Geometry check sheet. Reference: the model listing, model coordinates, mm. Face numbers are marked on the shaded views. A direction names the side the tool comes from. Round coordinates to 2 decimals unless told otherwise and drop trailing zeros. Order: outer loops, then holes, each group sorted by start corner. A loop starts at its lowest first (then second) coordinate and runs counter-clockwise, first axis right, second up. Notation, with made-up numbers: M 4,82.5 L 25,82.5 A18 ccw 25,116.5 Z; hole C 37,26.25 d1. An arc over 180 degrees is marked long. Return JSON: item names as keys, results as strings. Group by question number.
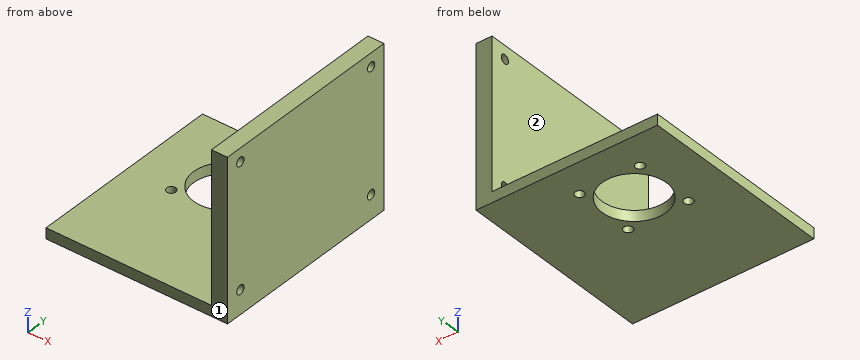
Solid Edge part; units mm, degrees
sketch "Sketch1" plane through (0, 0, 8) normal (0, 0, 1) x (1, 0, 0)
  line L0 (-28, -49) -> (40, -49)
  line L1 (40, -49) -> (40, 24)
  line L2 (40, 24) -> (-28, 24)
  line L3 (-28, 24) -> (-28, -49)
  circle A0 centre (0, 0) radius 12
  circle A1 centre (11.3137, 11.3137) radius 1.7
  circle A2 centre (-11.3137, 11.3137) radius 1.7
  circle A3 centre (-11.3137, -11.3137) radius 1.7
  circle A4 centre (11.3137, -11.3137) radius 1.7
extrude "ExtrudedProtrusion_1" add sketch "Sketch1" along normal blind 4
sketch "Sketch2" plane through (0, 0, 12) normal (0, 0, 1) x (1, 0, 0)
  line L0 (34, -49) -> (40, -49)
  line L1 (40, -49) -> (40, 24)
  line L2 (40, 24) -> (34, 24)
  line L3 (34, 24) -> (34, -49)
extrude "ExtrudedProtrusion_2" add sketch "Sketch2" along normal blind 56
sketch "Sketch3" plane through (34, 0, 0) normal (1, 0, 0) x (0, 1, 0)
  circle A0 centre (-43, 63) radius 1.7
  circle A1 centre (-43, 17) radius 1.7
  circle A2 centre (18, 63) radius 1.7
  circle A3 centre (18, 17) radius 1.7
extrude "ExtrudedCutout_1" cut sketch "Sketch3" along normal blind 6
Q1. Section check B-B on y = 18. Record the cut outline in (x, z).
Q2. Section check A-A on y = 0. Record the cut outline in (x, z).
Q3. Section check D-D on z = 17. Record the cut outline in (x, y).
Q4. Material ranges on line 1 along Z through (x, y) = (35.3, -43); line 2 along X through (y, z) = (-27, 15); line 3 along Z through (x, y) = (-20, -33), recorded low to high.
Q5. Depth check by flat-ended pin: pin 1 Ø10 at (x, y) = (22, -2.5) entering from +Z; pin 2 Ø1 at (y, z) = (-25, 34) entering from -X. Enter the tip coordinate at first touch or a pass-through.
Q6. Set-up check for the marked faces 1 and 2: record each of +Z, -Z, +X, -X, +Y, -Y from which the full face is reachable in a straight line by a thin tool's end or side.
Q7. Section check C-C on x = 0. Record the cut outline in (y, z).
Geometry check:
{
 "1": {"outline": "M -28,8 L 40,8 L 40,15.3 L 34,15.3 L 34,12 L -28,12 Z; M 34,18.7 L 40,18.7 L 40,61.3 L 34,61.3 Z; M 34,64.7 L 40,64.7 L 40,68 L 34,68 Z"},
 "2": {"outline": "M -28,8 L -12,8 L -12,12 L -28,12 Z; M 12,8 L 40,8 L 40,68 L 34,68 L 34,12 L 12,12 Z"},
 "3": {"outline": "M 34,-49 L 40,-49 L 40,-44.7 L 34,-44.7 Z; M 34,-41.3 L 40,-41.3 L 40,16.3 L 34,16.3 Z; M 34,19.7 L 40,19.7 L 40,24 L 34,24 Z"},
 "4": {"line 1": "z = 8 to 15.3, 18.7 to 61.3, 64.7 to 68", "line 2": "x = 34 to 40", "line 3": "z = 8 to 12"},
 "5": {"pin 1": "stops at z = 12", "pin 2": "stops at x = 34"},
 "6": {"face 1": "+Z, -Z, +X, -X, -Y", "face 2": "+Z, -X, +Y, -Y"},
 "7": {"outline": "M -49,8 L -12,8 L -12,12 L -49,12 Z; M 12,8 L 24,8 L 24,12 L 12,12 Z"}
}
